```python
from build123d import *

# Parameters (mm, degrees)
SKETCH1_W           = 130
SKETCH1_H           = 157
BOSS_EXTRUDE1_DEPTH = 100
CUT_EXTRUDE3_DEPTH  = 130
CUT_EXTRUDE7_DEPTH  = 157
SKETCH10_W          = 31
SKETCH10_H          = 58.139222378
CUT_EXTRUDE8_DEPTH  = 25
SKETCH11_W          = 93
SKETCH11_H          = 126
CUT_EXTRUDE9_DEPTH  = 97


with BuildPart() as part:
    # Sketch1 → Boss-Extrude1 (new body)
    with BuildSketch(Plane.XY):
        with Locations((89.509803922, -21.637254902)):
            Rectangle(SKETCH1_W, SKETCH1_H)
    extrude(amount=BOSS_EXTRUDE1_DEPTH)

    # Sketch3 → Cut-Extrude3 (cut)
    with BuildSketch(Plane(origin=(154.509803922, 0, 0), x_dir=(0, 0, -1), z_dir=(1, 0, 0))):
        with BuildLine():
            Line((-14, -97.137254902), (-56, -97.137254902))
            Line((-56, -97.137254902), (-56, -100.137254902))
            Line((-56, -100.137254902), (-100, -100.137254902))
            Line((-100, -100.137254902), (-100, -75.137254902))
            Line((-100, -75.137254902), (-14, -75.137254902))
            ThreePointArc((-14, -75.137254902), (-3, -86.137254902), (-14, -97.137254902))
        make_face()
    extrude(amount=-CUT_EXTRUDE3_DEPTH, mode=Mode.SUBTRACT)

    # Sketch9 → Cut-Extrude7 (cut)
    with BuildSketch(Plane(origin=(0, 56.862745098, 0), x_dir=(1, 0, 0), z_dir=(0, 1, 0))):
        with BuildLine():
            Line((27.509803922, -17), (27.509803922, -61.139222378))
            Line((27.509803922, -61.139222378), (24.509803922, -61.139222378))
            Line((24.509803922, -61.139222378), (24.509803922, -100))
            Line((24.509803922, -100), (55.509803922, -100))
            Line((55.509803922, -100), (55.509803922, -17))
            ThreePointArc((55.509803922, -17), (41.509803922, -3), (27.509803922, -17))
        make_face()
    extrude(amount=-CUT_EXTRUDE7_DEPTH, mode=Mode.SUBTRACT)

    # Sketch10 → Cut-Extrude8 (cut)
    with BuildSketch(Plane.XZ.offset(100.137254902)):
        with Locations((40.009803922, 32.069611189)):
            Rectangle(SKETCH10_W, SKETCH10_H)
    extrude(amount=-CUT_EXTRUDE8_DEPTH, mode=Mode.SUBTRACT)

    # Sketch11 → Cut-Extrude9 (cut)
    with BuildSketch(Plane(origin=(0, 0, 0), x_dir=(-1, 0, 0), z_dir=(0, 0, -1))):
        with Locations((-105.009803922, -9.137254902)):
            Rectangle(SKETCH11_W, SKETCH11_H)
    extrude(amount=-CUT_EXTRUDE9_DEPTH, mode=Mode.SUBTRACT)


solid = part.part
```
Build history of the part. All positions in model axes, mm. A direction names the side the tool comes from. Round coordinates to 2 decimals unless told otherwise and drop trailing zeros. Order: outer loops, then holes, each group sorted by start corner. A loop starts at its lowest first (then second) coordinate and runs counter-clockwise, first axis right, second up. Notation, with made-up numbers: (86.5, -3) -> (131.5, -3) arc R9 ccw to (131.5, 13) -> close; hole circle Ø9 at (47.5, 63). An arc over 180 degrees is marked (long way). Answer in a Markdown table with one row per item.
1) Pin check, flat tips, straight feed: P1, Ø4, axis at y = -96.5, z = 23, coming from the -X side; P2, Ø5, axis at x = 31, z = 32.5, coming from the -Y side; P3, Ø2.5, axis at x = 25.5, y = 9, coming from the +Z side; P4, Ø1.5, axis at x = 91.5, y = -99.5, coming from the +Z side. Stop position of each tip, or through.
Values:
| item | result |
|---|---|
| P1 | x = 55.51 |
| P2 | through |
| P3 | z = 61.14 |
| P4 | z = 56 |
2) Band-saw the part on D-D on x = 110.5. Give the cut face in (y, z), and give its area (3 significant figures).
Values:
| item | result |
|---|---|
| outline | (-100.14, 0) -> (-72.14, 0) -> (-72.14, 97) -> (53.86, 97) -> (53.86, 0) -> (56.86, 0) -> (56.86, 100) -> (-75.14, 100) -> (-75.14, 14) arc R11 cw to (-97.14, 14) -> (-97.14, 56) -> (-100.14, 56) -> close |
| area | 1,260 mm2 |
3) Band-saw the part on B-B on y = 18. Give the cut face in (x, z).
Values:
| item | result |
|---|---|
| outline | (24.51, 0) -> (58.51, 0) -> (58.51, 97) -> (151.51, 97) -> (151.51, 0) -> (154.51, 0) -> (154.51, 100) -> (55.51, 100) -> (55.51, 17) arc R14 cw to (27.51, 17) -> (27.51, 61.14) -> (24.51, 61.14) -> close |
4) Mould opens along Y. For faces 4 (the flat face through (103, -100.137, 28)), 5 (the flat face through (55.51, -8, 59)), 6 (the flat face through (106, 53.863, 48)) say: released by +Y, released by -Y, zero draft, split by the parting line, or undercut.
Values:
| item | result |
|---|---|
| face 4 | released by -Y |
| face 5 | zero draft |
| face 6 | undercut |
5) Wall check: L1, parallel to X at y = 43, z = 59; L2, parallel to Y at x = 91, z = 31.5; L3, parallel to Y at x = 110, z = 57.5. Give the ranges that are in metal, low to high.
Values:
| item | result |
|---|---|
| L1 | 24.51 to 27.51, 55.51 to 58.51, 151.51 to 154.51 |
| L2 | -100.14 to -97.14, -75.14 to -72.14, 53.86 to 56.86 |
| L3 | -75.14 to -72.14, 53.86 to 56.86 |
6) Which spindle directions (+Z, -Z, +X, -X, +Y, -Y) get a long thin tool onto all of the face, cutting with end or side? Do faces 1 (the flat face through (55.51, -98, 28)), 2 (the flat face through (151.51, -10, 48)), 3 (the flat face through (27.51, -8, 39)). Say none if no direction does.
Values:
| item | result |
|---|---|
| face 1 | +Z, -X, -Y |
| face 2 | -Z |
| face 3 | +Z, +Y, -Y |
7) Band-saw the part on A-A on z = 41. Give the cut face in (x, y), and give its area (3 significant figures).
Values:
| item | result |
|---|---|
| outline | (24.51, -75.14) -> (27.51, -75.14) -> (27.51, 56.86) -> (24.51, 56.86) -> close; (55.51, -100.14) -> (154.51, -100.14) -> (154.51, -97.14) -> (55.51, -97.14) -> close; (55.51, -75.14) -> (154.51, -75.14) -> (154.51, 56.86) -> (55.51, 56.86) -> close; hole (58.51, -72.14) -> (151.51, -72.14) -> (151.51, 53.86) -> (58.51, 53.86) -> close |
| area | 2,040 mm2 |
8) Band-saw the part on C-C on z = 74. Give the cut face in (x, y), and give its area (3 significant figures).
Values:
| item | result |
|---|---|
| outline | (55.51, -75.14) -> (154.51, -75.14) -> (154.51, 56.86) -> (55.51, 56.86) -> close; hole (58.51, -72.14) -> (151.51, -72.14) -> (151.51, 53.86) -> (58.51, 53.86) -> close |
| area | 1,350 mm2 |
